Geometry check sheet. Reference: the model listing, model coordinates, mm. A direction names the side the tool comes from. Coordinates: 2 decimals unless noted, no trailing zeros. Order: outer loops, then holes, each group sorted by start corner. A loop starts at its lowest first (then second) coordinate and runs counter-clockwise, first axis right, second up. Notation, with made-up numbers: (49.25, 37.5) - (107.25, 37.5) arc R17 cw to (107.25, 64.5) - close; hole circle Ø5 at (39.5, 19.5). An arc over 180 degrees is marked (long way). Return JSON: item names as keys, results as strings. Group by question number.
Item 1: Section check C-C on y = 1.15. Enter the section's corners in (x, z), then the cut area to 3 significant figures.
Item 2: Draft check along X on faces 1 (the flat face through (70, 2, -12.7)), 2 (the flat face through (80.01, 2, -38)), 3 (the flat face through (59.69, 2, -24)). Enter one of: pulls with the +X half, pulls with the -X half, needs draft (parallel to the pull), parting line crosses it, or undercut.
Item 3: Section check A-A on z = 28.5. Enter the section's corners in (x, y).
Item 4: Scan lines: probe 1 along X at (y, z) = (1.55, -34); probe 2 along Z at (x, y) = (46, 0.7); probe 3 along Z at (x, y) = (64, 0.3). Record each from-to range of solid material in increasing order.
Item 5: Section check B-B on x = 69. Enter the section's corners in (y, z).
Item 6: Gauge pin test, flat ends, axial feed: pin 1 (1.4 mm diameter, centred on y = 2.5, z = -3, fed in from -X); pin 2 (1.5 mm diameter, centred on x = 9, y = 3, fed in from -Z). Record the tip position at first contact, or that the pin passes through.
Item 7: Section check D-D on z = -11. Enter the section's corners in (x, y), then the cut area to 3 significant figures.
Item 8: Tool access check on faces 4 (the flat face through (-76, 2, -12.7)), 5 (the flat face through (40.64, 2, 0)), 6 (the flat face through (12.7, 2, -60)), 7 (the flat face through (0, 2, 56.134)). Record the directions out of +Z, -Z, +X, -X, +Y, -Y that give a thin tool (end or side, any length) a straight path to the whole face; none if there is none.
from build123d import *

# Parameters (mm, degrees)
BOSS_EXTRUDE1_DEPTH = 4.826
CUT_EXTRUDE1_DEPTH  = 4.826


with BuildPart() as part:
    # Sketch1 → Boss-Extrude1 (new body)
    with BuildSketch(Plane(origin=(0, 0, 0), x_dir=(1, 0, 0), z_dir=(0, 1, 0))):
        Polygon((-80.01, 63.5), (-12.7, 63.5), (-12.7, 56.134), (12.7, 56.134), (12.7, 63.5), (80.01, 63.5), (80.01, 12.7), (72.644, 12.7), (72.644, -12.7), (80.01, -12.7), (80.01, -63.5), (12.7, -63.5), (12.7, -56.134), (-12.7, -56.134), (-12.7, -63.5), (-80.01, -63.5), (-80.01, -12.7), (-72.644, -12.7), (-72.644, 12.7), (-80.01, 12.7), align=None)
    extrude(amount=BOSS_EXTRUDE1_DEPTH)

    # Sketch3 → Cut-Extrude1 (cut)
    with BuildSketch(Plane(origin=(0, 4.826, 0), x_dir=(1, 0, 0), z_dir=(0, 1, 0))):
        Polygon((59.69, -35.433), (40.64, -35.433), (40.64, 35.433), (59.69, 35.433), (59.69, 12.7), (72.644, 12.7), (72.644, -12.7), (59.69, -12.7), align=None)
    extrude(amount=-CUT_EXTRUDE1_DEPTH, mode=Mode.SUBTRACT)


solid = part.part
Computed:
{
 "1": {"outline": "(-80.01, -63.5) - (-12.7, -63.5) - (-12.7, -56.13) - (12.7, -56.13) - (12.7, -63.5) - (80.01, -63.5) - (80.01, -12.7) - (59.69, -12.7) - (59.69, -35.43) - (40.64, -35.43) - (40.64, 35.43) - (59.69, 35.43) - (59.69, 12.7) - (80.01, 12.7) - (80.01, 63.5) - (12.7, 63.5) - (12.7, 56.13) - (-12.7, 56.13) - (-12.7, 63.5) - (-80.01, 63.5) - (-80.01, 12.7) - (-72.64, 12.7) - (-72.64, -12.7) - (-80.01, -12.7) - close", "area": "17,900 mm²"},
 "2": {"face 1": "needs draft", "face 2": "pulls with the +X half", "face 3": "undercut"},
 "3": {"outline": "(-80.01, 0) - (40.64, 0) - (40.64, 4.83) - (-80.01, 4.83) - close; (59.69, 0) - (80.01, 0) - (80.01, 4.83) - (59.69, 4.83) - close"},
 "4": {"probe 1": "x = -80.01 to 40.64, 59.69 to 80.01", "probe 2": "z = -63.5 to -35.43, 35.43 to 63.5", "probe 3": "z = -63.5 to -12.7, 12.7 to 63.5"},
 "5": {"outline": "(0, -63.5) - (4.83, -63.5) - (4.83, -12.7) - (0, -12.7) - close; (0, 12.7) - (4.83, 12.7) - (4.83, 63.5) - (0, 63.5) - close"},
 "6": {"pin 1": "stops at x = -72.64", "pin 2": "stops at z = -56.13"},
 "7": {"outline": "(-72.64, 0) - (40.64, 0) - (40.64, 4.83) - (-72.64, 4.83) - close", "area": "547 mm²"},
 "8": {"face 4": "-X, +Y, -Y", "face 5": "+Y, -Y", "face 6": "-Z, +Y, -Y", "face 7": "+Z, +Y, -Y"}
}
